Geometry check sheet. Reference: the model listing, model coordinates, mm. Face numbers are marked on the shaded views. A direction names the side the tool comes from. Coordinates: 2 decimals unless noted, no trailing zeros. Write each loop counter-clockwise with the first axis right and the second up, starting at its lowest first coordinate (ties: lowest second). Pieces come first, ordered by that corner, then holes. Notation, with made-up numbers: M 3.5,55 L 32.5,55 A36 cw 32.5,94 Z; hole C 51,-28 d3. An arc over 180 degrees is marked long. Put each result on its own line as item: value. Start each with the question number.
1) Cross-section at A-A on z = 38.5. Record the cut outline in (x, y).
2) Cross-section at C-C on y = 10. Record the cut outline in (x, z), plus the area to 3 significant figures.
3) Mould release check, pull along Y, two halves, no side actions. Record for the marked faces 4, 5 and 6: released by +Y, released by -Y, zero draft, split by the parting line, or undercut.
4) Cross-section at D-D on z = -1. Record the cut outline in (x, y).
5) Set-up check for the marked faces 1, 2 and 3: record each of +Z, -Z, +X, -X, +Y, -Y from which the full face is reachable in a straight line by a thin tool's end or side.
6) Cross-section at B-B on x = -18. Record the cut outline in (y, z).
7) Gauge pin test, flat ends, axial feed: pin 1 (10 mm diameter, centred on x = -35.5, y = 49.5, fed in from +Z); pin 2 (1 mm diameter, centred on x = -17, y = 36, fed in from -Z); pin 3 (14 mm diameter, centred on y = 71.5, z = 18.5, fed in from -X). Record the tip position at first contact, or that the pin passes through.
8) Scan lines: line 1 along Y through (x, z) = (-37.5, 26); line 2 along Z through (x, y) = (-30, 54); line 3 along Z through (x, y) = (-27, 8). Record each from-to range of solid material in increasing order.
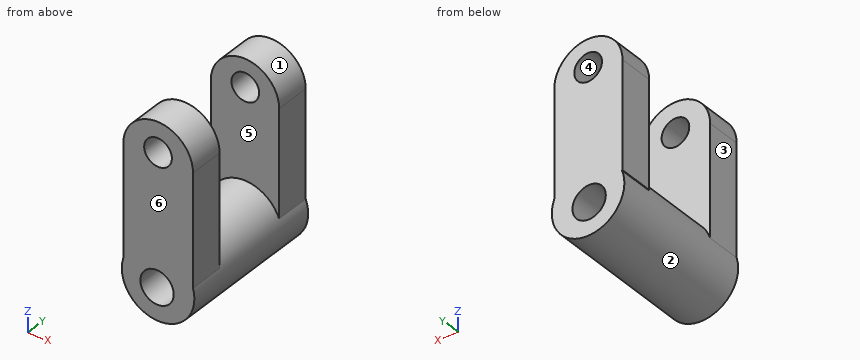
from build123d import *

# Parameters (mm, degrees)
F0_R      = 18.3156602834
F1_DEPTH  = 76.2
F2_W      = 35.1851196028
F2_H      = 56.3925905153
F3_DEPTH  = 17.78
F5_DEPTH  = 17.78
F7_DEPTH  = 17.78
F9_DEPTH  = 17.78
F10_R     = 6.9929791969
F11_DEPTH = 127
F12_R     = 8.4175574938
F13_DEPTH = 127


with BuildPart() as f1:
    # F0 (on Front) → F1 (new body)
    with BuildSketch(Plane.XZ):
        with Locations((-23.0617076159, -12.4766519293)):
            Circle(F0_R)
    extrude(amount=-F1_DEPTH)

    # F2 (on Front) → F3 (join)
    with BuildSketch(Plane.XZ):
        with Locations((-23.0149261188, 20.6049853005)):
            Rectangle(F2_W, F2_H)
    extrude(amount=-F3_DEPTH)

    # F4 (on face) → F5 (join)
    with BuildSketch(Plane(origin=(0, 76.2, 0), x_dir=(-1, 0, 0), z_dir=(0, 1, 0))):
        with BuildLine():
            Line((6.0013058485, 48.0782985687), (6.0013058485, -5.8128614799))
            ThreePointArc((6.0013058485, -5.8128614799), (23.0617076159, 5.8390083541), (40.1221093832, -5.8128614799))
            Line((40.1221093832, -5.8128614799), (40.4440611601, -5.8128614799))
            Line((40.4440611601, -5.8128614799), (40.4440611601, 48.0782985687))
            Line((40.4440611601, 48.0782985687), (6.0013058485, 48.0782985687))
        make_face()
    extrude(amount=-F5_DEPTH)

    # F6 (on face) → F7 (join)
    with BuildSketch(Plane.XZ):
        with BuildLine():
            Line((-40.6074859202, 48.8012805581), (-5.4223663174, 48.8012805581))
            ThreePointArc((-5.4223663174, 48.8012805581), (-23.0149261188, 66.3938403595), (-40.6074859202, 48.8012805581))
        make_face()
    extrude(amount=-F7_DEPTH)

    # F8 (on face) → F9 (join)
    with BuildSketch(Plane(origin=(0, 76.2, 0), x_dir=(-1, 0, 0), z_dir=(0, 1, 0))):
        with BuildLine():
            Line((6.0013058485, 48.0782985687), (40.4440611601, 48.0782985687))
            ThreePointArc((40.4440611601, 48.0782985687), (23.2226835043, 65.2996762245), (6.0013058485, 48.0782985687))
        make_face()
    extrude(amount=-F9_DEPTH)

    # F10 (on face) → F11 (cut)
    with BuildSketch(Plane(origin=(0, 76.2, 0), x_dir=(-1, 0, 0), z_dir=(0, 1, 0))):
        with Locations((23.0925008655, 51.4522157609)):
            Circle(F10_R)
    extrude(amount=-F11_DEPTH, mode=Mode.SUBTRACT)

    # F12 (on face) → F13 (cut)
    with BuildSketch(Plane(origin=(0, 76.2, 0), x_dir=(-1, 0, 0), z_dir=(0, 1, 0))):
        with Locations((23.5904790461, -14.580136165)):
            Circle(F12_R)
    extrude(amount=-F13_DEPTH, mode=Mode.SUBTRACT)


solid = f1.part
Answer key:
1. outline: M -40.61,0 L -5.42,0 L -5.42,17.78 L -40.61,17.78 Z; M -40.44,58.42 L -6,58.42 L -6,76.2 L -40.44,76.2 Z
2. outline: M -40.61,-7.22 A18.32 ccw long -5.42,-7.55 L -5.42,48.8 A17.59 ccw -40.61,48.8 Z; hole C -23.59,-14.58 d16.84; hole C -23.09,51.45 d13.99
2. area: 2,800 mm²
3. face 4: zero draft
3. face 5: undercut
3. face 6: released by -Y
4. outline: M -40.61,0 L -5.42,0 L -5.42,17.78 L -8.79,17.78 L -8.79,58.42 L -6,58.42 L -6,76.2 L -40.44,76.2 L -40.44,58.42 L -37.34,58.42 L -37.34,17.78 L -40.61,17.78 Z
5. face 1: +Z, +Y
5. face 2: none
5. face 3: +Z, -X, +Y, -Y
6. outline: M 0,-30.08 L 76.2,-30.08 L 76.2,-20.87 L 0,-20.87 Z; M 0,-8.29 L 76.2,-8.29 L 76.2,46.66 L 58.42,46.66 L 58.42,5.13 L 17.78,5.13 L 17.78,46.66 L 0,46.66 Z; M 0,56.24 L 17.78,56.24 L 17.78,65.66 L 0,65.66 Z; M 58.42,56.24 L 76.2,56.24 L 76.2,64.49 L 58.42,64.49 Z
7. pin 1: stops at z = 4.26
7. pin 2: stops at z = -29.93
7. pin 3: stops at x = -40.44
8. line 1: y = 0 to 17.78, 58.42 to 76.2
8. line 2: z = -29.43 to -20.04, -9.12 to 4.47
8. line 3: z = -30.36 to -22.28, -6.88 to 45.65, 57.25 to 65.94
